Verification items for the finished model (mm, model axes). Face numbers are marked on the shaded views. Coordinates: 2 decimals unless noted, no trailing zeros. Write each loop counter-clockwise with the first axis right and the second up, starting at its lowest first coordinate (ties: lowest second). Pieces come first, ordered by that corner, then holes. Notation, with made-up numbers: (-17.5, 30.25) -> (-13.5, 30.25) arc R33 ccw to (-13.5, 65.25) -> close; hole circle Ø2 at (87, 68). An arc over 180 degrees is marked (long way). Answer in a Markdown table with one row per item.
```python
from build123d import *

# Parameters (mm, degrees)
SKETCH_2_W           = 96.5
SKETCH_2_H           = 7
EXTRUDE_1_DEPTH      = 11
SKETCH_6_W           = 5
SKETCH_6_H           = 2.5
CUT_EXTRUDE_3_DEPTH  = 98.376845297
SKETCH_7_W           = 54.3
SKETCH_7_H           = 10
CUT_EXTRUDE_4_DEPTH  = 5
SKETCH_8_R           = 1.2
CUT_EXTRUDE_6_DEPTH  = 98.376845297
SKETCH_10_W          = 96.5
SKETCH_10_H          = 7
EXTRUDE_2_DEPTH      = 57
SKETCH_11_W          = 8
SKETCH_11_H          = 2
CUT_EXTRUDE_7_DEPTH  = 4
CHAMFER_1_SIZE       = 0.4
FILLET_1_R           = 3
SKETCH_12_W          = 54.2
SKETCH_12_H          = 84.200000954
CUT_EXTRUDE_8_DEPTH  = 5
CUT_EXTRUDE_9_DEPTH  = 119.15773356
CHAMFER_2_SIZE       = 2
CHAMFER_3_SIZE       = 0.6
SKETCH_17_W          = 13
SKETCH_17_H          = 8
CUT_EXTRUDE_10_DEPTH = 0.6
CUT_EXTRUDE_11_DEPTH = 4
CHAMFER_4_SIZE       = 1.5
SKETCH_19_R          = 2.05
CUT_EXTRUDE_12_DEPTH = 2
SKETCH_20_R          = 1.2
CUT_EXTRUDE_13_DEPTH = 119.15773356


with BuildPart() as part:
    # 草图2 → 凸台-拉伸1 (new body)
    with BuildSketch(Plane(origin=(0, 0, 0), x_dir=(0, 0, -1), z_dir=(1, 0, 0))):
        with Locations((48.25, 3.5)):
            Rectangle(SKETCH_2_W, SKETCH_2_H)
    extrude(amount=EXTRUDE_1_DEPTH)

    # 草图6 → 切除-拉伸3 (cut, through all)
    with BuildSketch(Plane(origin=(0, 0, -96.5), x_dir=(-1, 0, 0), z_dir=(0, 0, -1))):
        with Locations((-2.5, 3.75)):
            Rectangle(SKETCH_6_W, SKETCH_6_H)
        with Locations((-2.5, 1.25)):
            Rectangle(SKETCH_6_W, SKETCH_6_H)
    extrude(amount=-CUT_EXTRUDE_3_DEPTH, mode=Mode.SUBTRACT)

    # 草图7 → 切除-拉伸4 (cut)
    with BuildSketch(Plane.ZY):
        with Locations((-48.25, 9)):
            Rectangle(SKETCH_7_W, SKETCH_7_H)
    extrude(amount=-CUT_EXTRUDE_4_DEPTH, mode=Mode.SUBTRACT)

    # 草图8 → 切除-拉伸6 (cut, through all)
    with BuildSketch(Plane(origin=(0, 7, 0), x_dir=(1, 0, 0), z_dir=(0, 1, 0))):
        with Locations(Location((2.2, 15.75, 0), (0, 0, 270))):
            Circle(SKETCH_8_R)
        with Locations(Location((2.2, 80.75, 0), (0, 0, 270))):
            Circle(SKETCH_8_R)
    extrude(amount=-CUT_EXTRUDE_6_DEPTH, mode=Mode.SUBTRACT)

    # 草图10 → 凸台-拉伸2 (add)
    with BuildSketch(Plane(origin=(11, 0, 0), x_dir=(0, 0, -1), z_dir=(1, 0, 0))):
        with Locations((48.25, 3.5)):
            Rectangle(SKETCH_10_W, SKETCH_10_H)
    extrude(amount=EXTRUDE_2_DEPTH)

    # 草图11 → 切除-拉伸7 (cut)
    with BuildSketch(Plane.ZY):
        with Locations((-92.5, 6)):
            Rectangle(SKETCH_11_W, SKETCH_11_H)
        with Locations((-4, 6)):
            Rectangle(SKETCH_11_W, SKETCH_11_H)
    extrude(amount=-CUT_EXTRUDE_7_DEPTH, mode=Mode.SUBTRACT)

    # 倒角1
    chamfer_1_edges = [part.edges().sort_by_distance(p)[0] for p in [
        (4, 7, -92.5),
        (4, 7, -4),
    ]]
    chamfer(chamfer_1_edges, length=CHAMFER_1_SIZE)

    # 圆角1
    fillet_1_edges = [part.edges().sort_by_distance(p)[0] for p in [
        (68, 3.5, 0),
        (68, 3.5, -96.5),
    ]]
    fillet(fillet_1_edges, radius=FILLET_1_R)

    # 草图12 → 切除-拉伸8 (cut)
    with BuildSketch(Plane.XZ):
        with Locations((37.9, -48.499999523)):
            Rectangle(SKETCH_12_W, SKETCH_12_H)
    extrude(amount=-CUT_EXTRUDE_8_DEPTH, mode=Mode.SUBTRACT)

    # 草图16 → 切除-拉伸9 (cut, through all)
    with BuildSketch(Plane.XZ.offset(-5)):
        Polygon((45, -6.399999046), (63, -6.399999046), (63, -90.6), (12.8, -90.6), (12.8, -18.599999046), (45, -18.599999046), align=None)
    extrude(amount=-CUT_EXTRUDE_9_DEPTH, mode=Mode.SUBTRACT)

    # 倒角2
    chamfer_2_edges = [part.edges().sort_by_distance(p)[0] for p in [
        (45, 6, -18.599999046),
        (45, 6, -6.399999046),
        (63, 6, -6.399999046),
        (63, 6, -90.6),
        (12.8, 6, -90.6),
        (12.8, 6, -18.599999046),
    ]]
    chamfer(chamfer_2_edges, length=CHAMFER_2_SIZE)

    # 倒角3
    chamfer_3_edges = [part.edges().sort_by_distance(p)[0] for p in [
        (34.7, 7, -96.5),
        (67.121320344, 7, -95.621320344),
        (68, 7, -48.25),
        (67.121320344, 7, -0.878679656),
        (34.7, 7, 0),
        (62, 7, -89.6),
        (63, 7, -48.499999523),
        (62, 7, -7.399999046),
        (54, 7, -6.399999046),
        (46, 7, -7.399999046),
        (45, 7, -12.499999046),
        (44, 7, -17.599999046),
        (37.9, 7, -90.6),
        (13.8, 7, -89.6),
        (12.8, 7, -54.599999523),
        (13.8, 7, -19.599999046),
        (28.9, 7, -18.599999046),
    ]]
    chamfer(chamfer_3_edges, length=CHAMFER_3_SIZE)

    # 草图17 → 切除-拉伸10 (cut)
    with BuildSketch(Plane.XZ.offset(-5)):
        with Locations((26.1, -10.399999046)):
            Rectangle(SKETCH_17_W, SKETCH_17_H)
    extrude(amount=-CUT_EXTRUDE_10_DEPTH, mode=Mode.SUBTRACT)

    # 草图18 → 切除-拉伸11 (cut)
    with BuildSketch(Plane.XZ):
        Polygon((34.708261144, -6.399999046), (10.8, -6.399999046), (10.8, -63.25), (5, -63.25), (5, -33.25), (7.8, -33.25), (7.8, -1.2), (34.708261144, -1.2), align=None)
    extrude(amount=-CUT_EXTRUDE_11_DEPTH, mode=Mode.SUBTRACT)

    # 倒角4
    chamfer_4_edges = [part.edges().sort_by_distance(p)[0] for p in [
        (7.8, 2, -33.25),
        (7.8, 2, -1.2),
        (34.708261144, 2, -1.2),
    ]]
    chamfer(chamfer_4_edges, length=CHAMFER_4_SIZE)

    # 草图19 → 切除-拉伸12 (cut)
    with BuildSketch(Plane(origin=(0, 7, 0), x_dir=(1, 0, 0), z_dir=(0, 1, 0))):
        with Locations(Location((54.4, 3.4, 0), (0, 0, 270))):
            Circle(SKETCH_19_R)
        with Locations(Location((54.4, 93.3, 0), (0, 0, 270))):
            Circle(SKETCH_19_R)
    extrude(amount=-CUT_EXTRUDE_12_DEPTH, mode=Mode.SUBTRACT)

    # 草图20 → 切除-拉伸13 (cut, through all)
    with BuildSketch(Plane(origin=(0, 5, 0), x_dir=(1, 0, 0), z_dir=(0, 1, 0))):
        with Locations(Location((54.4, 3.4, 0), (0, 0, 270))):
            Circle(SKETCH_20_R)
        with Locations(Location((54.4, 93.3, 0), (0, 0, 270))):
            Circle(SKETCH_20_R)
    extrude(amount=-CUT_EXTRUDE_13_DEPTH, mode=Mode.SUBTRACT)


solid = part.part
```
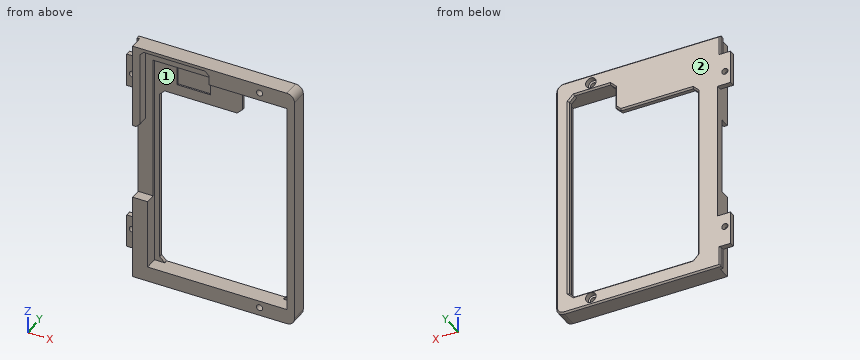
1. Sectioned sample at A-A, the plane z = -26. Record the cut outline in (x, y), and give its area (3 significant figures).
Findings below:
| item | result |
|---|---|
| outline | (5, 0) -> (7.8, 0) -> (7.8, 4) -> (10.8, 4) -> (10.8, 5) -> (12.8, 5) -> (12.8, 6.4) -> (12.2, 7) -> (5, 7) -> close; (63, 5) -> (65, 5) -> (65, 0) -> (68, 0) -> (68, 6.4) -> (67.4, 7) -> (63.6, 7) -> (63, 6.4) -> close |
| area | 57.1 mm² |
2. Material ranges on probe 1 along X at (y, z) = (5.5, -80.75); probe 2 along Z at (x, y) = (55, 4); probe 3 along X at (y, z) = (3, -27), recorded low to high. Write a range as from..to.
Findings below:
| item | result |
|---|---|
| probe 1 | x = 0..1, 3.4..12.8, 63..68 |
| probe 2 | z = -96.5..-94.34, -92.26..-90.6, -6.4..-4.44, -2.36..0 |
| probe 3 | x = 5..7.8, 65..68 |
3. Sectioned sample at C-C, the plane x = 2.2. Record the cut outline in (y, z).
Findings below:
| item | result |
|---|---|
| outline | (5, -88.5) -> (7, -88.5) -> (7, -81.95) -> (5, -81.95) -> close; (5, -79.55) -> (7, -79.55) -> (7, -75.4) -> (5, -75.4) -> close; (5, -21.1) -> (7, -21.1) -> (7, -16.95) -> (5, -16.95) -> close; (5, -14.55) -> (7, -14.55) -> (7, -8) -> (5, -8) -> close |
4. Go/stop test with flat-tipped pins: pin 1 (1.6 mm diameter, centred on x = 1.5, y = 6, fed in from -Z); pin 2 (3.5 mm diameter, centred on x = 53.5, z = -3.5, fed in from +Y); pin 3 (1.8 mm diameter, centred on y = 6, z = -5.5, fed in from -X); pin 4 (1.4 mm diameter, centred on x = 54.4, z = -3.4, fed in from -Y). Record where each tip stops, or that it passes through.
Findings below:
| item | result |
|---|---|
| pin 1 | stops at z = -88.5 |
| pin 2 | stops at y = 7 |
| pin 3 | stops at x = 4 |
| pin 4 | passes through |
5. Sectioned sample at D-D, the plane y = 2. Record the cut outline in (x, z), and give its area (3 significant figures).
Findings below:
| item | result |
|---|---|
| outline | (5, -96.5) -> (65, -96.5) arc R3 ccw to (68, -93.5) -> (68, -3) arc R3 ccw to (65, 0) -> (5, 0) -> (5, -33.25) -> (6.3, -33.25) -> (7.8, -31.75) -> (7.8, -2.7) -> (9.3, -1.2) -> (33.21, -1.2) -> (34.71, -2.7) -> (34.71, -6.4) -> (65, -6.4) -> (65, -90.6) -> (10.8, -90.6) -> (10.8, -63.25) -> (5, -63.25) -> close; hole circle Ø2.4 at (54.4, -93.3); hole circle Ø2.4 at (54.4, -3.4) |
| area | 1,110 mm² |
6. Release check for a two-part mould opening along X. For the marked faces 1 and 2 record: released by +X, released by -X, zero draft, split by the parting line, or undercut.
Findings below:
| item | result |
|---|---|
| face 1 | undercut |
| face 2 | zero draft |
7. Sectioned sample at B-B, the plane x = 31. Record the cut outline in (y, z), and give its area (3 significant figures).
Findings below:
| item | result |
|---|---|
| outline | (0, -96.5) -> (6.4, -96.5) -> (7, -95.9) -> (7, -91.2) -> (6.4, -90.6) -> (0, -90.6) -> close; (0, -1.2) -> (4, -1.2) -> (4, -6.4) -> (5.6, -6.4) -> (5.6, -14.4) -> (5, -14.4) -> (5, -18.6) -> (6.4, -18.6) -> (7, -18) -> (7, -0.6) -> (6.4, 0) -> (0, 0) -> close |
| area | 84.2 mm² |
